Verification items for this drawing (mm, ordinates from the low corner). A direction names the side the tool comes from. Round coordinates to 2 decimals unless told otherwise and drop trailing zeros. Write each loop counter-clockwise with the first axis right and the second up, starting at its lowest first coordinate (ties: lowest second). Pieces come first, ordered by that corner, then holes.
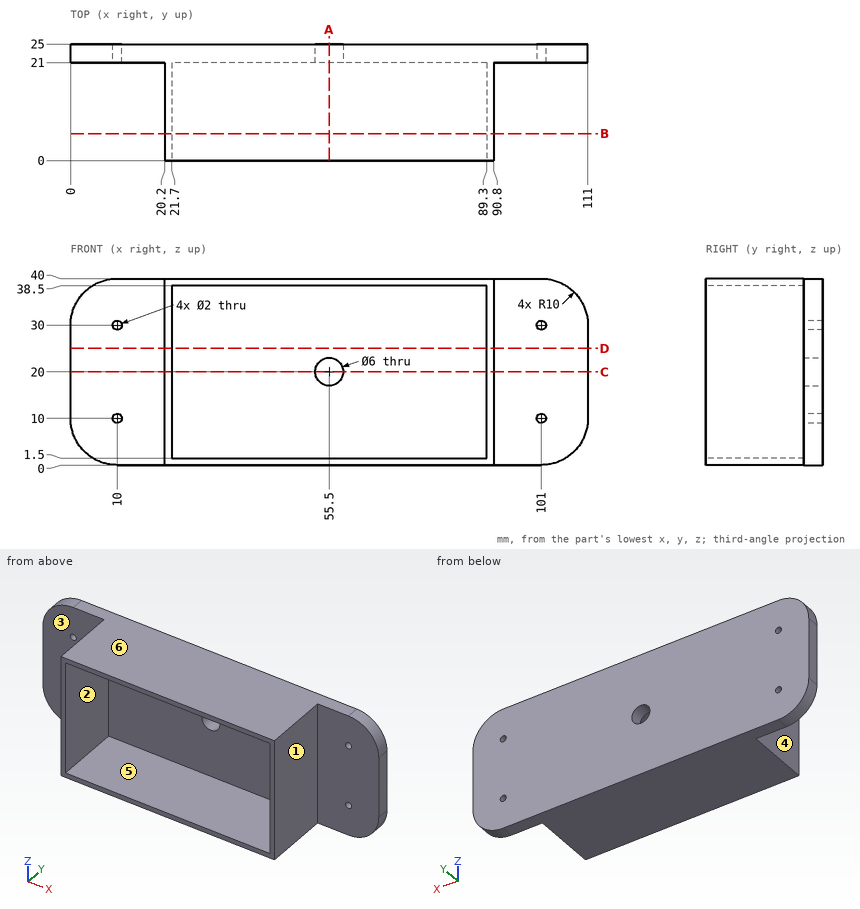
1. Section check C-C (z = 20). Record the cut outline in (x, y).
2. Section check A-A (x = 55.5). Record the cut outline in (y, z).
3. Release check for a two-part mould opening along Z. For the marked faces 4, 5 and 6 record: +Z half, -Z half, draft (parallel to the pull), parting line (faces both ways), or undercut.
4. Section check D-D (z = 25). Record the cut outline in (x, y).
5. Depth check by flat-ended pin: pin 1 Ø10.5 at (y, z) = (13, 11) entering from -X; pin 2 Ø10.5 at (y, z) = (11, 12.5) entering from +X; pin 3 Ø22 at (x, z) = (102, 23.5) entering from -Y. Enter the tip coordinate at first touch or a pass-through.
6. Scan lines: line 1 along Z through (x, y) = (10, 22.4); line 2 along X through (y, z) = (22.15, 10); line 3 along X through (y, z) = (14, 26.5). Record each from-to range of solid material in increasing order.
7. Section check B-B (y = 5.75). Record the cut outline in (x, z), plus the area to 3 significant figures.
8. Access from +Z, -Z, +X, -X, +Y, -Y to the whole of each face (thin tool, end or side, straight path). Record for the marked faces 1, 2 and 3.
Results below:
1. outline: (0, 21) - (20.2, 21) - (20.2, 0) - (21.7, 0) - (21.7, 21) - (52.5, 21) - (52.5, 25) - (0, 25) - close; (58.5, 21) - (89.3, 21) - (89.3, 0) - (90.8, 0) - (90.8, 21) - (111, 21) - (111, 25) - (58.5, 25) - close
2. outline: (0, 0) - (25, 0) - (25, 17) - (21, 17) - (21, 1.5) - (0, 1.5) - close; (0, 38.5) - (21, 38.5) - (21, 23) - (25, 23) - (25, 40) - (0, 40) - close
3. face 4: draft
3. face 5: undercut
3. face 6: +Z half
4. outline: (0, 21) - (20.2, 21) - (20.2, 0) - (21.7, 0) - (21.7, 21) - (89.3, 21) - (89.3, 0) - (90.8, 0) - (90.8, 21) - (111, 21) - (111, 25) - (0, 25) - close
5. pin 1: stops at x = 20.2
5. pin 2: stops at x = 90.8
5. pin 3: stops at y = 21
6. line 1: z = 0 to 9, 11 to 29, 31 to 40
6. line 2: x = 0 to 9, 11 to 100, 102 to 111
6. line 3: x = 20.2 to 21.7, 89.3 to 90.8
7. outline: (20.2, 0) - (90.8, 0) - (90.8, 40) - (20.2, 40) - close; hole (21.7, 1.5) - (89.3, 1.5) - (89.3, 38.5) - (21.7, 38.5) - close
7. area: 323 mm2
8. face 1: +Z, -Z, +X, -Y
8. face 2: -Y
8. face 3: +Z, -Z, -X, -Y
